Design review of the part built by this model. Coordinates are the model's own, in mm. Face numbers are marked on the shaded views. A direction names the side the tool comes from. Give positions to 0.01 mm unless a question says otherwise; leave off trailing zeros. Write each loop counter-clockwise with the first axis right and the second up, starting at its lowest first coordinate (ties: lowest second). Pieces come first, ordered by that corner, then holes. Notation, with made-up numbers: M 59,39.5 L 99,39.5 A35 ccw 99,78.5 Z; hole C -17,4.25 d7. An arc over 180 degrees is marked long. Write each question's results on one line, items separated by ' | '. Start each with the question number.
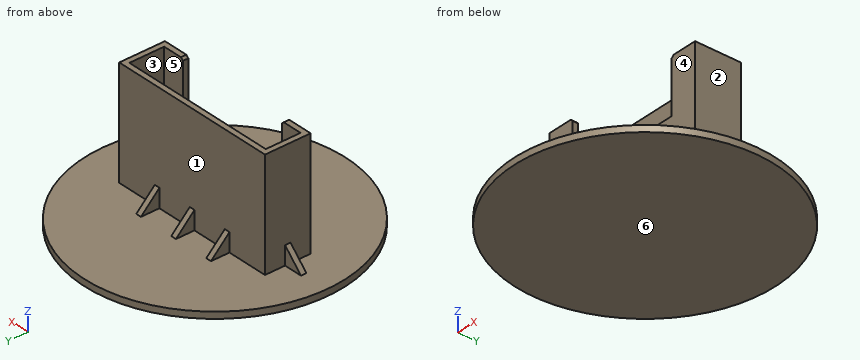
from build123d import *

# Parameters (mm, degrees)
F0_R         = 60
F0_W         = 8.5
F0_H         = 2.5
F0_W_2       = 2.5
F0_H_2       = 8.5
F2_DEPTH     = 3
F3_DEPTH     = 50
F4_T         = -2.5
F5_DEPTH     = 10
F6_T4_DEPTH  = 53.9336597593
F6_T10_DEPTH = 53.9336597593
F6_T16_DEPTH = 53.9336597593
F6_T22_DEPTH = 53.9336597593
F6_T28_DEPTH = 53.9336597593
F1_W         = 53
F1_H         = 50
F7_DEPTH     = 25
F8_SIZE      = 1


# Not quite as in the source:
# - a fillet or chamfer that OpenCascade refuses, or shapes differently, is made with other operations: its cross-section is extruded or revolved along the edge and cut away or added


with BuildPart() as f2:
    # F0 (on Top) → F2 (new body)
    with BuildSketch(Plane.XY):
        Circle(F0_R)
        Polygon((20, 10.5), (39, 10.5), (39, 1.25), (47.5, 1.25), (47.5, -1.25), (39, -1.25), (39, -10.5), (-39, -10.5), (-39, -1.25), (-47.5, -1.25), (-47.5, 1.25), (-39, 1.25), (-39, 10.5), (-20, 10.5), (-20, 19), (-17.5, 19), (-17.5, 10.5), (-1.25, 10.5), (-1.25, 19), (1.25, 19), (1.25, 10.5), (17.5, 10.5), (17.5, 19), (20, 19), align=None, mode=Mode.SUBTRACT)
        Polygon((39, 1.25), (39, 10.5), (20, 10.5), (17.5, 10.5), (1.25, 10.5), (-1.25, 10.5), (-17.5, 10.5), (-20, 10.5), (-39, 10.5), (-39, 1.25), (-39, -1.25), (-39, -10.5), (39, -10.5), (39, -1.25), align=None)
        with Locations((-43.25, 0)):
            Rectangle(F0_W, F0_H)
        with Locations((-18.75, 14.75)):
            Rectangle(F0_W_2, F0_H_2)
        with Locations((0, 14.75)):
            Rectangle(F0_W_2, F0_H_2)
        with Locations((18.75, 14.75)):
            Rectangle(F0_W_2, F0_H_2)
        with Locations((43.25, 0)):
            Rectangle(F0_W, F0_H)
    extrude(amount=-F2_DEPTH)

    # F0 (on Top) → F3 (join)
    with BuildSketch(Plane.XY):
        Polygon((39, 1.25), (39, 10.5), (20, 10.5), (17.5, 10.5), (1.25, 10.5), (-1.25, 10.5), (-17.5, 10.5), (-20, 10.5), (-39, 10.5), (-39, 1.25), (-39, -1.25), (-39, -10.5), (39, -10.5), (39, -1.25), align=None)
    extrude(amount=F3_DEPTH)

    # F4
    f4_openings = [f2.faces().sort_by_distance(p)[0] for p in [
        (0, 0, 50),
    ]]
    offset(amount=F4_T, openings=f4_openings, kind=Kind.INTERSECTION)

    # F0 (on Top) → F5 (join)
    with BuildSketch(Plane.XY):
        with Locations((18.75, 14.75)):
            Rectangle(F0_W_2, F0_H_2)
        with Locations((43.25, 0)):
            Rectangle(F0_W, F0_H)
        with Locations((0, 14.75)):
            Rectangle(F0_W_2, F0_H_2)
        with Locations((-18.75, 14.75)):
            Rectangle(F0_W_2, F0_H_2)
        with Locations((-43.25, 0)):
            Rectangle(F0_W, F0_H)
    extrude(amount=F5_DEPTH)

    # F6: chamfer of 10 on 5 edges, made by hand


with BuildPart() as f6_tool2:
    # F6_s3 → F6_t4 (new body)
    with BuildSketch(Plane.XZ.offset(26.9668298797)):
        Polygon((47.5, 0), (37.5, 10), (47.5, 10), align=None)
    extrude(amount=-F6_T4_DEPTH)

    split(bisect_by=Plane.XY, keep=Keep.TOP)

    split(bisect_by=Plane.YZ.offset(39), keep=Keep.TOP)


with BuildPart() as f2_1:
    add(f2.part)

    # F6_t1: cut F6_tool2
    add(f6_tool2.part, mode=Mode.SUBTRACT)


with BuildPart() as f6_tool8:
    # F6_s9 → F6_t10 (new body)
    with BuildSketch(Plane.YZ.offset(45.7168298797)):
        Polygon((19, 0), (9, 10), (19, 10), align=None)
    extrude(amount=-F6_T10_DEPTH)

    split(bisect_by=Plane.XY, keep=Keep.TOP)

    split(bisect_by=Plane.XZ.offset(-10.5), keep=Keep.BOTTOM)


with BuildPart() as f2_2:
    add(f2_1.part)

    # F6_t7: cut F6_tool8
    add(f6_tool8.part, mode=Mode.SUBTRACT)


with BuildPart() as f6_tool14:
    # F6_s15 → F6_t16 (new body)
    with BuildSketch(Plane.YZ.offset(26.9668298797)):
        Polygon((19, 0), (9, 10), (19, 10), align=None)
    extrude(amount=-F6_T16_DEPTH)

    split(bisect_by=Plane.XY, keep=Keep.TOP)

    split(bisect_by=Plane.XZ.offset(-10.5), keep=Keep.BOTTOM)


with BuildPart() as f2_3:
    add(f2_2.part)

    # F6_t13: cut F6_tool14
    add(f6_tool14.part, mode=Mode.SUBTRACT)


with BuildPart() as f6_tool20:
    # F6_s21 → F6_t22 (new body)
    with BuildSketch(Plane.YZ.offset(8.2168298797)):
        Polygon((19, 0), (9, 10), (19, 10), align=None)
    extrude(amount=-F6_T22_DEPTH)

    split(bisect_by=Plane.XY, keep=Keep.TOP)

    split(bisect_by=Plane.XZ.offset(-10.5), keep=Keep.BOTTOM)


with BuildPart() as f2_4:
    add(f2_3.part)

    # F6_t19: cut F6_tool20
    add(f6_tool20.part, mode=Mode.SUBTRACT)


with BuildPart() as f6_tool26:
    # F6_s27 → F6_t28 (new body)
    with BuildSketch(Plane.XZ.offset(-26.9668298797)):
        Polygon((-47.5, 0), (-37.5, 10), (-47.5, 10), align=None)
    extrude(amount=F6_T28_DEPTH)

    split(bisect_by=Plane.XY, keep=Keep.TOP)

    split(bisect_by=Plane.YZ.offset(-39), keep=Keep.BOTTOM)


with BuildPart() as f2_5:
    add(f2_4.part)

    # F6_t25: cut F6_tool26
    add(f6_tool26.part, mode=Mode.SUBTRACT)

    # F1 (on Front) → F7 (cut)
    with BuildSketch(Plane.XZ):
        with Locations((0, 50)):
            Rectangle(F1_W, F1_H)
    extrude(amount=F7_DEPTH, mode=Mode.SUBTRACT)

    # F8
    f8_edges = [f2_5.edges().sort_by_distance(p)[0] for p in [
        (-26.5, -9.25, 50),
        (26.5, -9.25, 50),
    ]]
    chamfer(f8_edges, length=F8_SIZE)


solid = f2_5.part
Q1. We need section A-A on z = 18. Write out the cut boundary in (x, y).
Q2. We need section B-B on z = 29. Write out the cut boundary in (x, y), and give its area (4 significant figures).
Q3. We need section C-C on y = 14. Write out the cut boundary in (x, z).
Q4. The part is to be moulded in two halves that separate along Y. For the marked faces 1, 2, 3 and 4, say which applies: pulls with the +Y half, pulls with the -Y half, needs draft (parallel to the pull), parting line crosses it, or undercut.
Q5. Wall thickness on line 1 along Y through (x, z) = (-8.5, 9); line 2 along X through (y, z) = (-4.5, 6); line 3 along Y through (x, z) = (18.5, 47): over which ranges is each line inside the solid? List them lowest first. Write a range as from..to.
Q6. We need section D-D on x = -8. Write out the cut boundary in (y, z).
Q7. For the marked faces 5 and 6, list the 3-axis set-ups (+Z, -Z, +X, -X, +Y, -Y) from which the entire face can be reached by the end or side of a thin tool; tool diameter is ignored.
Q8. For pin 1 Ø15 at (x, z) = (3.5, 21.5) entering from +Y; pin 2 Ø2.5 at (y, z) = (13.5, 4) entering from -X; pin 3 Ø25 at (x, z) = (-14.5, 21.5) entering from -Y; pin 4 Ø4 at (y, z) = (16, 6.5) entering from -X, all flat-tipped, find the tip position at first contact; note any pin that passes through.
Answer sheet:
1) outline: M -39,-10.5 L 39,-10.5 L 39,10.5 L -39,10.5 Z; hole M -36.5,-8 L 36.5,-8 L 36.5,8 L -36.5,8 Z
2) outline: M -39,-10.5 L -26.5,-10.5 L -26.5,-8 L -36.5,-8 L -36.5,8 L 36.5,8 L 36.5,-8 L 26.5,-8 L 26.5,-10.5 L 39,-10.5 L 39,10.5 L -39,10.5 Z | area: 337.5 mm^2
3) outline: M -58.34,-3 L 58.34,-3 L 58.34,0 L 20,0 L 20,5 L 17.5,5 L 17.5,0 L 1.25,0 L 1.25,5 L -1.25,5 L -1.25,0 L -17.5,0 L -17.5,5 L -20,5 L -20,0 L -58.34,0 Z
4) face 1: pulls with the +Y half | face 2: needs draft | face 3: undercut | face 4: pulls with the -Y half
5) line 1: -10.5..-8, 8..10.5 | line 2: -39..-36.5, 36.5..39 | line 3: 8..10.5
6) outline: M -59.46,-3 L 59.46,-3 L 59.46,0 L 10.5,0 L 10.5,50 L 8,50 L 8,-0.5 L -8,-0.5 L -8,25 L -10.5,25 L -10.5,0 L -59.46,0 Z
7) face 5: +Z | face 6: -Z, +X, -X, +Y, -Y
8) pin 1: y = 10.5 | pin 2: x = -20 | pin 3: y = -10.5 | pin 4: through
